```python
from build123d import *

# Parameters (mm, degrees)
SKETCH1_6_R         = 2
SKETCH1_6_R_2       = 3.915
BOSS_EXTRUDE3_DEPTH = 3


with BuildPart() as part:
    # Sketch1_6 → Boss-Extrude3 (new body)
    with BuildSketch(Plane(origin=(0, 0, 0), x_dir=(1, 0, 0), z_dir=(0, 1, 0))):
        Polygon((106.296761578, 32.295700632), (106.296761578, 6.055177331), (112.296761578, 6.055177331), (112.296761578, -26.969822669), (152.296761578, -26.969822669), (152.296761578, 32.295700632), align=None)
        with Locations(Location((142.296761578, -18.969822669, 0), (0, 0, 270))):
            Circle(SKETCH1_6_R, mode=Mode.SUBTRACT)
        with Locations(Location((118.466761578, 17.055177331, 0), (0, 0, 270))):
            Circle(SKETCH1_6_R_2, mode=Mode.SUBTRACT)
        with Locations(Location((137.296761578, 4.305177331, 0), (0, 0, 270))):
            Circle(SKETCH1_6_R_2, mode=Mode.SUBTRACT)
    extrude(amount=BOSS_EXTRUDE3_DEPTH)


solid = part.part
```
Verification items for the finished model (mm, model axes). A direction names the side the tool comes from. Coordinates: 2 decimals unless noted, no trailing zeros. Write each loop counter-clockwise with the first axis right and the second up, starting at its lowest first coordinate (ties: lowest second). Pieces come first, ordered by that corner, then holes. Notation, with made-up numbers: M 41.5,-27.5 L 88.5,-27.5 A25 ccw 88.5,-10.5 Z; hole C -13.75,30.25 d8. An arc over 180 degrees is marked long. Answer as a JSON object with one key per item and string values. Group by question number.
(1) Release check for a two-part mould opening along Z. For faces 3 (the face through (129, 0, -3)), 4 (the face through (140.52, 1.48, 19.89)), 5 (the face through (132, 1, 26.97)) record: +Z half, -Z half, draft (parallel to the pull), parting line (faces both ways), or undercut.
(2) Cross-section at C-C, the plane y = 2.25. Record the cut outline in (x, z) (3 decimals).
(3) Cross-section at B-B, the plane x = 120. Record the cut outline in (y, z).
(4) Material ranges on line 1 (X direction, y = 0.3, z = 1); line 2 (X direction, y = 2.25, z = -19.5); line 3 (Z direction, x = 139, y = 0.6), recorded low to high.
(5) Cross-section at D-D, the plane x = 111. Record the cut outline in (y, z).
(6) Cross-section at A-A, the plane z = 19.5. Record the cut outline in (x, y), and give its area (3 significant figures).
(7) Gauge pin test, flat ends, axial feed: pin 1 (10 mm diameter, centred on x = 111, z = 10.5, fed in from -Y); pin 2 (0.9 mm diameter, centred on x = 110.5, y = 1, fed in from +Z); pin 3 (0.9 mm diameter, centred on y = 1, z = 5.5, fed in from -X). Record the tip position at first contact, or that the pin passes through.
(8) Tool access check on faces 1 (the face through (109, 1, -6.055)), 2 (the face through (152.297, 1, -2)). Record the directions out of +Z, -Z, +X, -X, +Y, -Y that give a thin tool (end or side, any length) a straight path to the whole face; none if there is none.
Reply:
{
 "1": {"face 3": "draft", "face 4": "undercut", "face 5": "+Z half"},
 "2": {"outline": "M 106.297,-32.296 L 152.297,-32.296 L 152.297,26.97 L 112.297,26.97 L 112.297,-6.055 L 106.297,-6.055 Z; hole C 118.467,-17.055 d7.83; hole C 137.297,-4.305 d7.83; hole C 142.297,18.97 d4"},
 "3": {"outline": "M 0,-32.3 L 3,-32.3 L 3,-20.66 L 0,-20.66 Z; M 0,-13.45 L 3,-13.45 L 3,26.97 L 0,26.97 Z"},
 "4": {"line 1": "112.3 to 152.3", "line 2": "106.3 to 115.41, 121.52 to 152.3", "line 3": "-32.3 to -7.83, -0.78 to 26.97"},
 "5": {"outline": "M 0,-32.3 L 3,-32.3 L 3,-6.06 L 0,-6.06 Z"},
 "6": {"outline": "M 112.3,0 L 140.37,0 L 140.37,3 L 112.3,3 Z; M 144.23,0 L 152.3,0 L 152.3,3 L 144.23,3 Z", "area": "108 mm²"},
 "7": {"pin 1": "y = 0", "pin 2": "z = -6.06", "pin 3": "x = 112.3"},
 "8": {"face 1": "+Z, -X, +Y, -Y", "face 2": "+Z, -Z, +X, +Y, -Y"}
}
